Geometry check sheet. Reference: the model listing, model coordinates, mm. Face numbers are marked on the shaded views. A direction names the side the tool comes from. Round coordinates to 2 decimals unless told otherwise and drop trailing zeros. Order: outer loops, then holes, each group sorted by start corner. A loop starts at its lowest first (then second) coordinate and runs counter-clockwise, first axis right, second up.
(1) Release check for a two-part mould opening along Z. For the marked faces 5, 6, 7 and 8 record: +Z half, -Z half, draft (parallel to the pull), parting line (faces both ways), or undercut.
(2) Set-up check for the marked faces 1, 2, 3 and 4: record each of +Z, -Z, +X, -X, +Y, -Y from which the full face is reachable in a straight line by a thin tool's end or side.
(3) Sectioned sample at C-C (x = -88.35). Record the boundary of the cut face in (y, z).
(4) Go/stop test with flat-tipped pins: pin 1 (12.5 mm diameter, centred on x = 130, z = 4, fed in from -Y); pin 2 (8 mm diameter, centred on y = 10, z = -9.5, fed in from -X); pin 3 (11 mm diameter, centred on x = 124, y = 9, fed in from -Z); pin 4 (6.5 mm diameter, centred on y = 3.5, z = 8, fed in from -X). Record where each tip stops, or that it passes through.
(5) Sectioned sample at A-A (y = 6). Record the boundary of the cut face in (x, z), plus the area to 3 significant figures.
(6) Material ranges on line 1 along Z through (x, y) = (-63.5, 4.5); line 2 along Z through (x, y) = (49, 1.5); line 3 along X through (y, z) = (20.75, 3.25), recorded low to high.
(7) Sectioned sample at B-B (x = 9.5). Record the boundary of the cut face in (y, z).
(8) Sectioned sample at D-D (y = 17). Record the boundary of the cut face in (x, z).
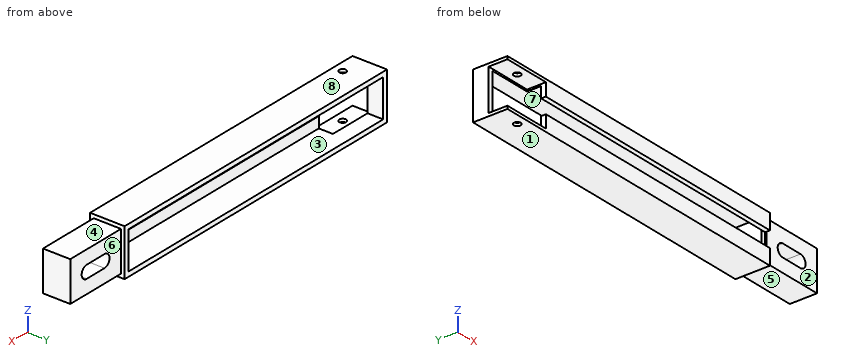
from build123d import *

# Parameters (mm, degrees)
SKETCH1_W           = 207
SKETCH1_H           = 30
BOSS_EXTRUDE1_DEPTH = 22
SHELL1_T            = -3
SKETCH2_W           = 207
SKETCH2_H           = 10
CUT_EXTRUDE1_DEPTH  = 3
SKETCH3_W           = 30.3
SKETCH3_H           = 26.3
CUT_EXTRUDE2_DEPTH  = 12
SKETCH4_R           = 2.2
CUT_EXTRUDE3_DEPTH  = 110.982953225
SKETCH5_W           = 25.4
SKETCH5_H           = 17.4
BOSS_EXTRUDE2_DEPTH = 40
CUT_EXTRUDE4_DEPTH  = 146.620534266


with BuildPart() as part:
    # Sketch1 → Boss-Extrude1 (new body)
    with BuildSketch(Plane(origin=(0, 0, 0), x_dir=(1, 0, 0), z_dir=(0, 1, 0))):
        Rectangle(SKETCH1_W, SKETCH1_H)
    extrude(amount=BOSS_EXTRUDE1_DEPTH)

    # Shell1
    shell1_openings = [part.faces().sort_by_distance(p)[0] for p in [
        (0, 22, 0),
    ]]
    offset(amount=SHELL1_T, openings=shell1_openings, kind=Kind.INTERSECTION)

    # Sketch2 → Cut-Extrude1 (cut)
    with BuildSketch(Plane(origin=(0, 0, 0), x_dir=(-1, 0, 0), z_dir=(0, -1, 0))):
        Rectangle(SKETCH2_W, SKETCH2_H)
    extrude(amount=-CUT_EXTRUDE1_DEPTH, mode=Mode.SUBTRACT)

    # Sketch3 → Cut-Extrude2 (cut)
    with BuildSketch(Plane(origin=(0, 0, 0), x_dir=(-1, 0, 0), z_dir=(0, -1, 0))):
        with Locations((88.35, 0)):
            Rectangle(SKETCH3_W, SKETCH3_H)
    extrude(amount=-CUT_EXTRUDE2_DEPTH, mode=Mode.SUBTRACT)

    # Sketch4 → Cut-Extrude3 (cut, through all)
    with BuildSketch(Plane.XY.offset(15)):
        with Locations((-88.35, 6)):
            Circle(SKETCH4_R)
    extrude(amount=-CUT_EXTRUDE3_DEPTH, mode=Mode.SUBTRACT)

    # Sketch5 → Boss-Extrude2 (add)
    with BuildSketch(Plane(origin=(103.5, 0, 0), x_dir=(0, 0, -1), z_dir=(1, 0, 0))):
        with Locations((0, 11)):
            Rectangle(SKETCH5_W, SKETCH5_H)
    extrude(amount=BOSS_EXTRUDE2_DEPTH)

    # Sketch6 → Cut-Extrude4 (cut, through all)
    with BuildSketch(Plane(origin=(0, 19.7, 0), x_dir=(1, 0, 0), z_dir=(0, 1, 0))):
        with BuildLine():
            Line((116.5, 4), (130.5, 4))
            ThreePointArc((130.5, 4), (134.5, 0), (130.5, -4))
            Line((130.5, -4), (116.5, -4))
            ThreePointArc((116.5, -4), (112.5, 0), (116.5, 4))
        make_face()
    extrude(amount=-CUT_EXTRUDE4_DEPTH, mode=Mode.SUBTRACT)


solid = part.part
Answer below:
1. face 5: -Z half
1. face 6: draft
1. face 7: undercut
1. face 8: +Z half
2. face 1: -Z, +X, -X, +Y, -Y
2. face 2: +Z, -Z, +X, -Y
2. face 3: +Y
2. face 4: +Z, +X, +Y, -Y
3. outline: (0, -15) - (3.8, -15) - (3.8, -13.15) - (0, -13.15) - close; (0, 13.15) - (3.8, 13.15) - (3.8, 15) - (0, 15) - close; (8.2, -15) - (22, -15) - (22, -12) - (12, -12) - (12, -13.15) - (8.2, -13.15) - close; (8.2, 13.15) - (12, 13.15) - (12, 12) - (22, 12) - (22, 15) - (8.2, 15) - close
4. pin 1: stops at y = 2.3
4. pin 2: stops at x = -103.5
4. pin 3: stops at z = -12.7
4. pin 4: stops at x = -73.2
5. outline: (-103.5, -15) - (-90.55, -15) - (-90.55, -13.15) - (-103.5, -13.15) - close; (-103.5, 13.15) - (-90.55, 13.15) - (-90.55, 15) - (-103.5, 15) - close; (-86.15, -15) - (103.5, -15) - (103.5, -12.7) - (143.5, -12.7) - (143.5, 12.7) - (103.5, 12.7) - (103.5, 15) - (-86.15, 15) - (-86.15, 13.15) - (-73.2, 13.15) - (-73.2, 12) - (100.5, 12) - (100.5, -12) - (-73.2, -12) - (-73.2, -13.15) - (-86.15, -13.15) - close; hole (116.5, -4) - (130.5, -4) arc R4 ccw to (130.5, 4) - (116.5, 4) arc R4 ccw to start
5. area: 2,080 mm2
6. line 1: z = -15 to -12, 12 to 15
6. line 2: z = -15 to -5, 5 to 15
6. line 3: x = -103.5 to -100.5, 100.5 to 103.5
7. outline: (0, -15) - (22, -15) - (22, -12) - (3, -12) - (3, -5) - (0, -5) - close; (0, 5) - (3, 5) - (3, 12) - (22, 12) - (22, 15) - (0, 15) - close
8. outline: (-103.5, -15) - (103.5, -15) - (103.5, -12.7) - (143.5, -12.7) - (143.5, 12.7) - (103.5, 12.7) - (103.5, 15) - (-103.5, 15) - close; hole (-100.5, -12) - (100.5, -12) - (100.5, 12) - (-100.5, 12) - close; hole (116.5, -4) - (130.5, -4) arc R4 ccw to (130.5, 4) - (116.5, 4) arc R4 ccw to start
